```python
from build123d import *

# Parameters (mm, degrees)
F0_R     = 3
F1_DEPTH = 25
F3_D     = 6.8
F3_DEPTH = 12
F3_TIP   = 2.0429261047


with BuildPart() as f1:
    # F0 (on Front) → F1 (new body)
    with BuildSketch(Plane.XZ):
        with BuildLine():
            Line((70, 50), (-70, 50))
            ThreePointArc((-70, 50), (-73.5355339059, 48.5355339059), (-75, 45))
            Line((-75, 45), (-75, -45))
            ThreePointArc((-75, -45), (-73.5355339059, -48.5355339059), (-70, -50))
            Line((-70, -50), (70, -50))
            ThreePointArc((70, -50), (73.5355339059, -48.5355339059), (75, -45))
            Line((75, -45), (75, 45))
            ThreePointArc((75, 45), (73.5355339059, 48.5355339059), (70, 50))
        make_face()
        with Locations((-37.5, -15)):
            Circle(F0_R, mode=Mode.SUBTRACT)
        with Locations((37.5, -15)):
            Circle(F0_R, mode=Mode.SUBTRACT)
        with Locations((-37.5, 15)):
            Circle(F0_R, mode=Mode.SUBTRACT)
        with Locations((37.5, 15)):
            Circle(F0_R, mode=Mode.SUBTRACT)
    extrude(amount=F1_DEPTH)

    # F3
    with Locations(Plane.XZ.offset(25)):
        with Locations((0, 0), (0, 50)):
            Hole(F3_D / 2, depth=F3_DEPTH)
            with Locations((0, 0, -(F3_DEPTH + F3_TIP / 2))):  # 118° drill point
                Cone(0, F3_D / 2, F3_TIP, mode=Mode.SUBTRACT)


solid = f1.part
```
Geometry check sheet. Reference: the model listing, model coordinates, mm. A direction names the side the tool comes from. Coordinates: 2 decimals unless noted, no trailing zeros. Order: outer loops, then holes, each group sorted by start corner. A loop starts at its lowest first (then second) coordinate and runs counter-clockwise, first axis right, second up. Notation, with made-up numbers: M 56.25,36 L 102.25,36 A21 ccw 102.25,73 Z; hole C 47,19.25 d8. An arc over 180 degrees is marked long. One line per question, with ' | ' between items. Start each with the question number.
Item 1: Cross-section at A-A on x = 37.5. Enter the section's corners in (y, z), then the cut area to 3 significant figures.
Item 2: Gauge pin test, flat end, axial feed: pin 1 (5 mm diameter, centred on x = -37.5, z = 15, fed in from -Y). Record the tip position at first contact, or that the pin passes through.
Item 3: Material ranges on L1, parallel to Z at x = 37.5, y = -10; L2, parallel to Z at x = 0, y = -13; L3, parallel to Z at x = 36, y = -20.75, recorded low to high. Write a range as [from, to].
Item 4: Draft check along Z on faces 4 (the cylindrical face through (-74, -12, -48)), 5 (the cylindrical face through (34.5, -12.3, -14.9)), 6 (the flat face through (75, -12, -1)). Enter one of: pulls with the +Z half, pulls with the -Z half, needs draft (parallel to the pull), parting line crosses it, or undercut.
Item 5: Set-up check for faces 1 (the cylindrical face through (-40.5, -12.3, 15.1)), 2 (the cylindrical face through (0.74, -18.92, -3.32)), 3 (the cylindrical face through (0.1, -18.9, 46.6)): record each of +Z, -Z, +X, -X, +Y, -Y from which the full face is reachable in a straight line by a thin tool's end or side.
Item 6: Cross-section at B-B on z = -15. Enter the section's corners in (x, y).
Findings:
1) outline: M -25,-50 L 0,-50 L 0,-18 L -25,-18 Z; M -25,-12 L 0,-12 L 0,12 L -25,12 Z; M -25,18 L 0,18 L 0,50 L -25,50 Z | area: 2,200 mm²
2) pin 1: passes through
3) L1: z = [-50, -18], [-12, 12], [18, 50] | L2: z = [-50, -3.4], [3.4, 46.6] | L3: z = [-50, -17.6], [-12.4, 12.4], [17.6, 50]
4) face 4: pulls with the -Z half | face 5: undercut | face 6: needs draft
5) face 1: +Y, -Y | face 2: -Y | face 3: +Z, -Y
6) outline: M -75,-25 L -40.5,-25 L -40.5,0 L -75,0 Z; M -34.5,-25 L 34.5,-25 L 34.5,0 L -34.5,0 Z; M 40.5,-25 L 75,-25 L 75,0 L 40.5,0 Z
